Geometry: final body of the model. Coordinates: model frame, mm. Face numbers are marked on the shaded views. A direction names the side the tool comes from. Coordinates: 2 decimals unless noted, no trailing zeros. Order: outer loops, then holes, each group sorted by start corner. A loop starts at its lowest first (then second) coordinate and runs counter-clockwise, first axis right, second up. Notation, with made-up numbers: (-35.5, 66.25) -> (1.5, 66.25) arc R26 cw to (1.5, 82.25) -> close; hole circle Ø11 at (78, -7). An arc over 180 degrees is marked (long way). Answer in a Markdown table with one row per item. Add a question column.
1) Section query C-C on x = -13. Return the cut outline in (y, z).
2) Set-up query: the marked faces 1, 2 and 3. Return all of +Z, -Z, +X, -X, +Y, -Y with unobstructed straight access to the full face (end or side cutting, diameter ignored); none if empty.
3) Ray query, line 1 (Y direction, x = 0, z = 9.1); line 2 (Y direction, x = 0, z = -1.7); line 3 (Y direction, x = -23, z = 9). Return the intervals inside material, ascending. Write a range as from..to.
4) Contact query for flat-ended pins moving along their axis: P1, Ø2.5, axis at x = -23, z = 4.5, coming from the +Y side; P2, Ø1.2, axis at x = -23.38, y = -13.5, coming from the -Z side; P3, Ø1.8, axis at x = 0.5, z = 2, coming from the +Y side; P4, Ø2.5, axis at x = -23.38, y = 13.5, coming from the -Z side. Output: stop coordinate, or through.
5) Section query A-A on y = 0. Return the cut outline in (x, z).
6) Section query D-D on z = -1.75. Return the cut outline in (x, y).
7) Pull-direction query (Y, two-part tool) for the marked faces 4, 5, 6 and 7; classes: +Y half, -Y half, draft (parallel to the pull), parting line (faces both ways), or undercut.
8) Section query B-B on z = 10.25. Return the cut outline in (x, y).
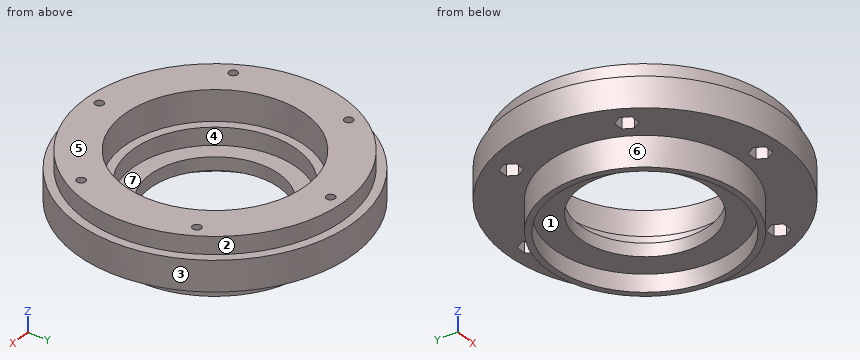
```python
from build123d import *

# Parameters (mm, degrees)
SKETCH_1_R          = 32
SKETCH_1_R_2        = 19
EXTRUDE_1_DEPTH     = 4
SKETCH_2_R          = 32
SKETCH_2_R_2        = 21
EXTRUDE_2_DEPTH     = 7
SKETCH_3_R          = 1
CUT_EXTRUDE_1_DEPTH = 47.572524089
CUT_EXTRUDE_2_DEPTH = 6
SKETCH_5_R          = 22.45
SKETCH_5_R_2        = 15
EXTRUDE_3_DEPTH     = 7
SKETCH_6_R          = 21.05
CUT_EXTRUDE_3_DEPTH = 4
CUT_EXTRUDE_START   = -4
SKETCH_7_R          = 32
SKETCH_7_R_2        = 30
CUT_EXTRUDE_4_DEPTH = 4


with BuildPart() as part:
    # 草图1 → 凸台-拉伸1 (new body)
    with BuildSketch(Plane.XY):
        Circle(SKETCH_1_R)
        Circle(SKETCH_1_R_2, mode=Mode.SUBTRACT)
    extrude(amount=EXTRUDE_1_DEPTH)

    # 草图2 → 凸台-拉伸2 (add)
    with BuildSketch(Plane.XY.offset(4)):
        Circle(SKETCH_2_R)
        Circle(SKETCH_2_R_2, mode=Mode.SUBTRACT)
    extrude(amount=EXTRUDE_2_DEPTH)

    # 草图3 → 切除-拉伸1 (cut, through all)
    with BuildSketch(Plane.XY.offset(11)):
        with Locations((0, 27)):
            Circle(SKETCH_3_R)
        with Locations((23.382685902, 13.5)):
            Circle(SKETCH_3_R)
        with Locations((23.382685902, -13.5)):
            Circle(SKETCH_3_R)
        with Locations((0, -27)):
            Circle(SKETCH_3_R)
        with Locations((-23.382685902, -13.5)):
            Circle(SKETCH_3_R)
        with Locations((-23.382685902, 13.5)):
            Circle(SKETCH_3_R)
    extrude(amount=-CUT_EXTRUDE_1_DEPTH, mode=Mode.SUBTRACT)

    # 草图4 → 切除-拉伸2 (cut)
    with BuildSketch(Plane(origin=(0, 0, 0), x_dir=(-1, 0, 0), z_dir=(0, 0, -1))):
        Polygon((21.073284825, 13.5), (22.227985364, 11.5), (24.537386441, 11.5), (25.692086979, 13.5), (24.537386441, 15.5), (22.227985364, 15.5), align=None)
        Polygon((-1.154700538, 25), (1.154700538, 25), (2.309401077, 27), (1.154700538, 29), (-1.154700538, 29), (-2.309401077, 27), align=None)
        Polygon((22.227985364, -11.5), (21.073284825, -13.5), (22.227985364, -15.5), (24.537386441, -15.5), (25.692086979, -13.5), (24.537386441, -11.5), align=None)
        Polygon((1.154700538, -25), (-1.154700538, -25), (-2.309401077, -27), (-1.154700538, -29), (1.154700538, -29), (2.309401077, -27), align=None)
        Polygon((-21.073284825, -13.5), (-22.227985364, -11.5), (-24.537386441, -11.5), (-25.692086979, -13.5), (-24.537386441, -15.5), (-22.227985364, -15.5), align=None)
        Polygon((-22.227985364, 11.5), (-21.073284825, 13.5), (-22.227985364, 15.5), (-24.537386441, 15.5), (-25.692086979, 13.5), (-24.537386441, 11.5), align=None)
    extrude(amount=-CUT_EXTRUDE_2_DEPTH, mode=Mode.SUBTRACT)

    # 草图5 → 凸台-拉伸3 (add)
    with BuildSketch(Plane(origin=(0, 0, 0), x_dir=(-1, 0, 0), z_dir=(0, 0, -1))):
        with Locations(Location((0, 0, 0), (0, 0, 180))):
            Circle(SKETCH_5_R)
        Circle(SKETCH_5_R_2, mode=Mode.SUBTRACT)
    extrude(amount=EXTRUDE_3_DEPTH)

    # 草图6 → 切除-拉伸3 (cut)
    with BuildSketch(Plane(origin=(0, 0, -7), x_dir=(-1, 0, 0), z_dir=(0, 0, -1))):
        Circle(SKETCH_6_R)
    extrude(amount=-CUT_EXTRUDE_3_DEPTH, mode=Mode.SUBTRACT)

    # 草图7 → 切除-拉伸4 (cut)
    with BuildSketch(Plane.XY.offset(11).offset(CUT_EXTRUDE_START)):
        Circle(SKETCH_7_R)
        Circle(SKETCH_7_R_2, mode=Mode.SUBTRACT)
    extrude(amount=CUT_EXTRUDE_4_DEPTH, mode=Mode.SUBTRACT)


solid = part.part
```
Result:
| question | item | result |
|---|---|---|
| 1 | outline | (-29.24, 0) -> (-18.3, 0) -> (-18.3, -7) -> (-16.56, -7) -> (-16.56, -3) -> (-7.48, -3) -> (-7.48, 0) -> (-13.86, 0) -> (-13.86, 4) -> (-16.49, 4) -> (-16.49, 11) -> (-27.04, 11) -> (-27.04, 7) -> (-29.24, 7) -> close; (7.48, -3) -> (16.56, -3) -> (16.56, -7) -> (18.3, -7) -> (18.3, 0) -> (29.24, 0) -> (29.24, 7) -> (27.04, 7) -> (27.04, 11) -> (16.49, 11) -> (16.49, 4) -> (13.86, 4) -> (13.86, 0) -> (7.48, 0) -> close |
| 2 | face 1 | -Z |
| 2 | face 2 | +Z |
| 2 | face 3 | +Z, -Z |
| 3 | line 1 | -30..-28, -26..-21, 21..26, 28..30 |
| 3 | line 2 | -22.45..-15, 15..22.45 |
| 3 | line 3 | -19.26..-14.42, -12.58..12.58, 14.42..19.26 |
| 4 | P1 | y = 23.47 |
| 4 | P2 | through |
| 4 | P3 | y = 32 |
| 4 | P4 | z = 6 |
| 5 | outline | (-32, 0) -> (-22.45, 0) -> (-22.45, -7) -> (-21.05, -7) -> (-21.05, -3) -> (-15, -3) -> (-15, 0) -> (-19, 0) -> (-19, 4) -> (-21, 4) -> (-21, 11) -> (-30, 11) -> (-30, 7) -> (-32, 7) -> close; (15, -3) -> (21.05, -3) -> (21.05, -7) -> (22.45, -7) -> (22.45, 0) -> (32, 0) -> (32, 7) -> (30, 7) -> (30, 11) -> (21, 11) -> (21, 4) -> (19, 4) -> (19, 0) -> (15, 0) -> close |
| 6 | outline | circle Ø44.9 at (0, 0); hole circle Ø30 at (0, 0) |
| 7 | face 4 | undercut |
| 7 | face 5 | draft |
| 7 | face 6 | parting line |
| 7 | face 7 | undercut |
| 8 | outline | circle Ø60 at (0, 0); hole circle Ø2 at (-23.38, -13.5); hole circle Ø2 at (-23.38, 13.5); hole circle Ø42 at (0, 0); hole circle Ø2 at (0, -27); hole circle Ø2 at (0, 27); hole circle Ø2 at (23.38, -13.5); hole circle Ø2 at (23.38, 13.5) |
